```python
from build123d import *

# Parameters (mm, degrees)
SKETCH_1_R          = 12.5
SKETCH_1_R_2        = 3
EXTRUDE_1_DEPTH     = 10
SKETCH_2_R          = 1.6
CUT_EXTRUDE_4_DEPTH = 12.5
SKETCH_3_R          = 5
EXTRUDE_2_DEPTH     = 3
SKETCH_4_R          = 18
EXTRUDE_3_DEPTH     = 2.5
FILLET_1_R          = 1
SKETCH_5_R          = 1
CUT_EXTRUDE_5_DEPTH = 3
FILLET_2_R          = 1


with BuildPart() as part:
    # 草图1 → 凸台-拉伸1 (new body)
    with BuildSketch(Plane(origin=(0, 0, 0), x_dir=(1, 0, 0), z_dir=(0, 1, 0))):
        with Locations(Location((0, 0, 0), (0, 0, 270))):
            Circle(SKETCH_1_R)
        with Locations(Location((0, 0, 0), (0, 0, 270))):
            Circle(SKETCH_1_R_2, mode=Mode.SUBTRACT)
    extrude(amount=EXTRUDE_1_DEPTH)

    # 草图2 → 切除-拉伸4 (cut, symmetric)
    with BuildSketch(Plane.XY):
        with Locations((0, 5)):
            Circle(SKETCH_2_R)
    extrude(amount=CUT_EXTRUDE_4_DEPTH, both=True, mode=Mode.SUBTRACT)

    # 草图3 → 凸台-拉伸2 (add)
    with BuildSketch(Plane(origin=(0, 10, 0), x_dir=(1, 0, 0), z_dir=(0, 1, 0))):
        with BuildLine():
            Line((1.160714286, 24.97304031), (280.557142857, 11.987059349))
            ThreePointArc((280.557142857, 11.987059349), (292, 0), (280.557142857, -11.987059349))
            Line((280.557142857, -11.987059349), (1.160714286, -24.97304031))
            ThreePointArc((1.160714286, -24.97304031), (-25, 0), (1.160714286, 24.97304031))
        make_face()
        with Locations(Location((280, 0, 0), (0, 0, 270))):
            Circle(SKETCH_3_R, mode=Mode.SUBTRACT)
        with Locations(Location((120, 0, 0), (0, 0, 270))):
            Circle(SKETCH_3_R, mode=Mode.SUBTRACT)
    extrude(amount=EXTRUDE_2_DEPTH)

    # 草图4 → 凸台-拉伸3 (add)
    with BuildSketch(Plane.XZ.offset(-10)):
        with Locations(Location((0, 0, 0), (0, 0, 270))):
            Circle(SKETCH_4_R)
    extrude(amount=EXTRUDE_3_DEPTH)

    # 圆角1
    fillet_1_edges = [part.edges().sort_by_distance(p)[0] for p in [
        (0, 7.5, 18),
    ]]
    fillet(fillet_1_edges, radius=FILLET_1_R)

    # 草图5 → 切除-拉伸5 (cut)
    with BuildSketch(Plane.XZ.offset(-10)):
        with Locations((120, 0)):
            Circle(SKETCH_5_R)
        Polygon((24.0562108, 4), (111.937742252, 4), (12.545084957, 20.439591429), align=None)
        Polygon((12.545084957, -20.439591429), (24.0562108, -4), (111.937742252, -4), align=None)
    extrude(amount=-CUT_EXTRUDE_5_DEPTH, mode=Mode.SUBTRACT)

    # 圆角2
    fillet_2_edges = [part.edges().sort_by_distance(p)[0] for p in [
        (24.0562108, 11.5, 4),
        (12.545084957, 11.5, 20.439591429),
        (111.937742252, 11.5, 4),
        (111.937742252, 11.5, -4),
        (12.545084957, 11.5, -20.439591429),
        (24.0562108, 11.5, -4),
    ]]
    fillet(fillet_2_edges, radius=FILLET_2_R)


solid = part.part
```
Can you work these out from the model? Positions are in its coordinate system, mm. A direction names the side the tool comes from. Coordinates: 2 decimals unless noted, no trailing zeros. Write each loop counter-clockwise with the first axis right and the second up, starting at its lowest first coordinate (ties: lowest second). Pieces come first, ordered by that corner, then holes. Notation, with made-up numbers: M -29.75,24.25 L 9.25,24.25 A25 ccw 9.25,53.25 Z; hole C -9,4 d9. An arc over 180 degrees is marked long. Write item = value, one per line. Start each with the question number.
Q1. If we section it at B-B, the plane x = 120: Write out the boundary of the cut face in (y, z).
Q2. On a 3-axis mill with a long thin cutter (end or side, diameter ignored), from which of +Z, -Z, +X, -X, +Y, -Y can I reach the whole of each face in a straight line? I mean faces 1 (the face through (0, 7.5, 0)), 2 (the face through (-3, 0, 3)), 3 (the face through (18.765, 11.479, 11.557)). Say none if no direction works.
Q3. If I drill on L1, parallel to X at y = 5.25, z = 0; L2, parallel to Z at x = 44.5, y = 12; L3, parallel to Y at x = 0, z = 9, over which ranges is the centre line in solid material (lowest first)? Write a range as [from, to].
Q4. If we section it at A-A, the plane x = 88: Write out the boundary of the cut face in (y, z).
Q5. If we section it at C-C, the plane x = 195: Write out the boundary of the cut face in (y, z).
Q6. Thinking about a two-plate mould opening in X: for faces 4 (the face through (3.755, 3.698, 11.923)), 5 (the face through (138.9, 11.48, -18.57)), 6 (the face through (58, 11.48, 12.92)), which applies, released by +X, released by -X, zero draft, split by the parting line, or undercut?
Q7. I'm going to push flat-ended pins straight in: pin 1 (3 mm diameter, centred on x = 187, z = 17, fed in from -Y); pin 2 (1.5 mm diameter, centred on x = 48.5, y = 11, fed in from -Z); pin 3 (10 mm diameter, centred on x = -2, z = 8, fed in from -Y); pin 4 (0.9 mm diameter, centred on x = 49, y = 11.5, fed in from +Z). Where does each tip first touch, or does it pass through?
Q8. If we section it at D-D, the plane x = 162: Write out the boundary of the cut face in (y, z), then the cut area to 3 significant figures.
Check sheet entries:
q1.outline = M 10,-19.45 L 13,-19.45 L 13,-5 L 10,-5 Z; M 10,5 L 13,5 L 13,19.45 L 10,19.45 Z
q2.face_1 = -Y
q2.face_2 = +Z, -Z, +X, -X, -Y
q2.face_3 = +Y, -Y
q3.L1 = [-12.5, -3], [3, 12.5]
q3.L2 = [-22.96, -15.15], [-4, 4], [15.15, 22.96]
q3.L3 = [0, 3.4], [6.6, 13]
q4.outline = M 10,-20.94 L 13,-20.94 L 13,-7.96 L 10,-7.96 Z; M 10,-4 L 13,-4 L 13,4 L 10,4 Z; M 10,7.96 L 13,7.96 L 13,20.94 L 10,20.94 Z
q5.outline = M 10,-15.96 L 13,-15.96 L 13,15.96 L 10,15.96 Z
q6.face_4 = split by the parting line
q6.face_5 = released by +X
q6.face_6 = undercut
q7.pin_1 = 10
q7.pin_2 = -22.81
q7.pin_3 = 0
q7.pin_4 = 22.77
q8.outline = M 10,-17.5 L 13,-17.5 L 13,17.5 L 10,17.5 Z
q8.area = 105 mm²
